Verification items for the finished model (mm, model axes). Round coordinates to 2 decimals unless told otherwise and drop trailing zeros. Write each loop counter-clockwise with the first axis right and the second up, starting at its lowest first coordinate (ties: lowest second). Pieces come first, ordered by that corner, then holes. Notation, with made-up numbers: M 66,40 L 114,40 A19 ccw 114,55 Z; hole C -4,-21.5 d6. An arc over 180 degrees is marked long. Answer in a Markdown table with one row per item. Add a question column.
1. Material ranges on probe 1 along Y at (x, z) = (7, -0.5); probe 2 along X at (y, z) = (14, -1.4); probe 3 along Y at (x, z) = (-22.5, -0.55), recorded low to high.
2. Go/stop test with flat-tipped pins: pin 1 Ø1 at (x, z) = (-5, -0.5) entering from -Y; pin 2 Ø0.5 at (y, z) = (-13.5, -1) entering from +X. Record where each tip stops, or that it passes through.
3. Sectioned sample at A-A on x = -9.05. Record the cut outline in (y, z).
4. Sectioned sample at B-B on z = -1.4. Record the cut outline in (x, y), plus the area to 3 significant figures.
5. Sectioned sample at C-C on x = -15.5. Record the cut outline in (y, z), plus the area to 3 significant figures.
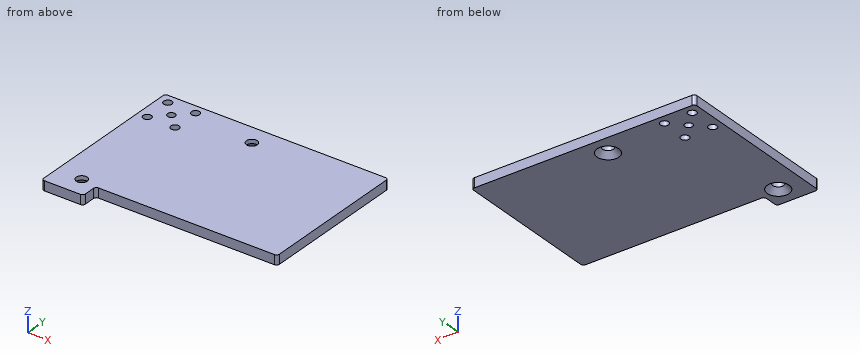
Autodesk Inventor part; units mm, degrees
ref_plane "YZ Plane" through (0, 0, 0) normal (1, 0, 0) x (0, 1, 0)
ref_plane "XZ Plane" through (0, 0, 0) normal (0, 1, 0) x (-1, 0, 0)
ref_plane "XY Plane" through (0, 0, 0) normal (0, 0, 1) x (1, 0, 0)
sketch "Boceto1" plane through (0, 0, 0) normal (0, 0, 1) x (1, 0, 0)
  line L0 (-26, 17) -> (26, 17)
  line L1 (26, 17) -> (26, -17)
  line L2 (26, -17) -> (-26, -17)
  line L3 (-26, -17) -> (-26, 17)
  line L4 (-26, 17) -> (26, -17) construction
  line L5 (26, 17) -> (-26, -17) construction
  point P0 (0, 0)
  dimension "d0" = 52
  dimension "d1" = 34
extrude "Extrusión1" add sketch "Boceto1" against normal blind 1.742
fillet "Empalme1" radius 0.5 4 edges at (26, 17, -0.871) (-26, 17, -0.871) (-26, -17, -0.871) (26, -17, -0.871)
sketch "Boceto2" plane through (0, 0, 0) normal (0, 0, 1) x (1, 0, 0)
  line L0 (25.5, 17) -> (-25.5, 17)
  line L1 (26, 16.5) -> (26, -16.5)
  line L2 (25.5, -17) -> (-25.5, -17) construction
  line L3 (23, -17) -> (-20, -17)
  line L4 (-20, -17) -> (-20, -12.2)
  line L5 (-20, -12.2) -> (23, -12.2)
  line L6 (23, -12.2) -> (23, -17)
  point P0 (0, 0)
  dimension "d13" = 3
  dimension "d14" = 4.8
  dimension "d15" = 43
extrude "Extrusión2" cut sketch "Boceto2" against normal through all
sketch "Boceto3" plane through (0, 0, -1.742) normal (0, 0, -1) x (-1, 0, 0)
  arc A0 (26, 16.5) -> (25.5, 17) centre (25.5, 16.5) ccw
  line L0 (26, -16.5) -> (26, 16.5)
  arc A1 (25.5, -17) -> (26, -16.5) centre (25.5, -16.5) ccw
  line L1 (25.5, 17) -> (27.6, 17)
  line L2 (27.6, 17) -> (27.6, -17)
  line L3 (27.6, -17) -> (25.5, -17)
  point P0 (0, 0)
  dimension "d10" = 1.6
extrude "Extrusión3" add sketch "Boceto3" against normal up to surface (1.742 mm away)
sketch "Boceto4" plane through (0, 0, 0) normal (0, 0, 1) x (1, 0, 0)
  line L0 (-27.6, 17) -> (25.5, 17) construction
  arc A0 (26, 16.5) -> (25.5, 17) centre (25.5, 16.5) ccw construction
  line L1 (26, 16.5) -> (26, -16.5) construction
  line L2 (25.5, -17) -> (23, -17) construction
  arc A1 (25.5, -17) -> (26, -16.5) centre (25.5, -16.5) ccw construction
  line L3 (23, -12.2) -> (23, -17) construction
  line L4 (-20, -12.2) -> (23, -12.2) construction
  line L5 (26, 17) -> (22.8, 17)
  line L6 (22.8, 17) -> (22.8, -17)
  line L7 (22.8, -17) -> (26, -17)
  line L8 (26, -17) -> (26, 17)
  point P0 (0, 0)
  dimension "d16" = 3.2
  dimension "d17" = 34
extrude "Extrusión4" cut sketch "Boceto4" against normal up to surface (1.742 mm away)
sketch "Boceto5" plane through (0, 0, 0) normal (0, 0, 1) x (1, 0, 0)
  line L0 (-27.6, 17) -> (22.8, 17)
  line L1 (22.8, 17) -> (13.2, 17)
  line L2 (13.2, 17) -> (13.2, -12.2)
  line L3 (13.2, -12.2) -> (22.8, -12.2)
  line L4 (22.8, -12.2) -> (22.8, 17)
  point P0 (0, 0)
  point P1 (22.8, -12.2)
  dimension "d20" = 9.6
extrude "Extrusión5" cut sketch "Boceto5" against normal up to surface (1.742 mm away)
fillet "Empalme2" radius 1 3 edges at (-27.6, -17, -0.871) (-27.6, 17, -0.871) (13.2, 17, -0.871)
sketch "Boceto8" plane through (0, 0, -1.742) normal (0, 0, -1) x (-1, 0, 0)
  line L0 (20, -17) -> (26.6, -17)
  line L1 (20, -12.2) -> (20, -17)
  point P0 (0, 0)
  point P1 (22.95, -11.638)
  dimension "d54" = 5.362
  dimension "d55" = 2.95
hole "Agujero3" at (-22.95, -11.638, -1.742) direction (0, 0, 1) diameter 2 end through all countersink diameter 4 countersink angle 90
sketch "Boceto9" plane through (0, 0, -1.742) normal (0, 0, -1) x (-1, 0, 0)
  line L0 (-13.2, 16) -> (-13.2, -12.2)
  line L1 (26.6, 17) -> (-12.2, 17)
  point P0 (0, 0)
  point P1 (9.05, 11.638)
  dimension "d52" = 22.25
  dimension "d53" = 5.362
hole "Agujero4" at (-9.05, 11.638, -1.742) direction (0, 0, 1) diameter 2 end through all countersink diameter 4 countersink angle 90
sketch "Boceto10" plane through (0, 0, -1.742) normal (0, 0, -1) x (-1, 0, 0)
  line L0 (20.7601, 13.5399) -> (25.8399, 13.5399) construction
  line L1 (25.8399, 13.5399) -> (25.8399, 8.4601) construction
  line L2 (25.8399, 8.4601) -> (20.7601, 8.4601) construction
  line L3 (20.7601, 8.4601) -> (20.7601, 13.5399) construction
  line L4 (20.7601, 13.5399) -> (25.8399, 8.4601) construction
  line L5 (26.6, 17) -> (-12.2, 17) construction
  line L6 (27.6, -16) -> (27.6, 16) construction
  circle A0 centre (20.7601, 13.5399) radius 0.75
  circle A1 centre (25.8399, 13.5399) radius 0.75
  circle A2 centre (20.7601, 8.4601) radius 0.75
  circle A3 centre (25.8399, 8.4601) radius 0.75
  circle A4 centre (23.3, 11) radius 0.7
  point P0 (0, 0)
  dimension "d56" = 7.184
  dimension "d57" = 45
  dimension "d58" = 6
  dimension "d59" = 4.3
  dimension "d60" = 1.5
  dimension "d61" = 1.5
  dimension "d62" = 1.5
  dimension "d63" = 1.5
  dimension "d64" = 1.4
extrude "Extrusión6" cut sketch "Boceto10" against normal up to surface (1.742 mm away)
fillet "Empalme3" radius 0.5 1 edges at (13.2, -12.2, -0.871)
fillet "Empalme4" radius 0.5 2 edges at (-20, -17, -0.871) (-20, -12.2, -0.871)
sketch "Boceto11" plane through (0, 0, -1.742) normal (0, 0, -1) x (-1, 0, 0)
  line L0 (-13.2, 17) -> (27.6, 17)
  line L1 (27.6, 17) -> (27.6, 15.258)
  line L2 (27.6, 15.258) -> (-13.2, 15.258)
  line L3 (-13.2, 15.258) -> (-13.2, 17)
  line L4 (-13.2, 16) -> (-13.2, -11.7)
  line L5 (27.6, -16) -> (27.6, 16)
  line L6 (20, -15.258) -> (27.6, -15.258)
  line L7 (27.6, -15.258) -> (27.6, -17)
  line L8 (27.6, -17) -> (20, -17)
  line L9 (20, -17) -> (20, -15.258)
  line L10 (20, -12.7) -> (20, -16.5)
  line L11 (20.5, -17) -> (26.6, -17)
  point P0 (0, 0)
  point P1 (26.6, 17)
  dimension "d69" = 1.742
  dimension "d70" = 1.742
extrude "Extrusión7" cut sketch "Boceto11" against normal up to surface (1.742 mm away)
fillet "Empalme5" radius 0.5 4 edges at (13.2, 15.258, -0.871) (-27.6, 15.258, -0.871) (-20, -15.258, -0.871) (-27.6, -15.258, -0.871)
properties part number "hw_DAA - PCB MicroSD" material "PCB"
Geometry check:
| question | item | result |
|---|---|---|
| 1 | probe 1 | y = -12.2 to 15.26 |
| 1 | probe 2 | x = -27.6 to -26.43, -25.25 to -21.35, -20.17 to 13.2 |
| 1 | probe 3 | y = -15.26 to -12.53, -10.74 to 15.26 |
| 2 | pin 1 | stops at y = -12.2 |
| 2 | pin 2 | stops at x = -20 |
| 3 | outline | M -12.2,-1.74 L 9.64,-1.74 L 10.64,-0.74 L 10.64,0 L -12.2,0 Z; M 12.64,-0.74 L 13.64,-1.74 L 15.26,-1.74 L 15.26,0 L 12.64,0 Z |
| 4 | outline | M -27.6,-14.76 A0.5 ccw -27.1,-15.26 L -20.5,-15.26 A0.5 ccw -20,-14.76 L -20,-12.7 A0.5 cw -19.5,-12.2 L 12.7,-12.2 A0.5 ccw 13.2,-11.7 L 13.2,14.76 A0.5 ccw 12.7,15.26 L -27.1,15.26 A0.5 ccw -27.6,14.76 Z; hole C -25.84,8.46 d1.5; hole C -25.84,13.54 d1.5; hole C -22.95,-11.64 d3.32; hole C -23.3,11 d1.4; hole C -20.76,8.46 d1.5; hole C -20.76,13.54 d1.5; hole C -9.05,11.64 d3.32 |
| 4 | area | 1,120 mm2 |
| 5 | outline | M -12.2,-1.74 L 15.26,-1.74 L 15.26,0 L -12.2,0 Z |
| 5 | area | 47.8 mm2 |
